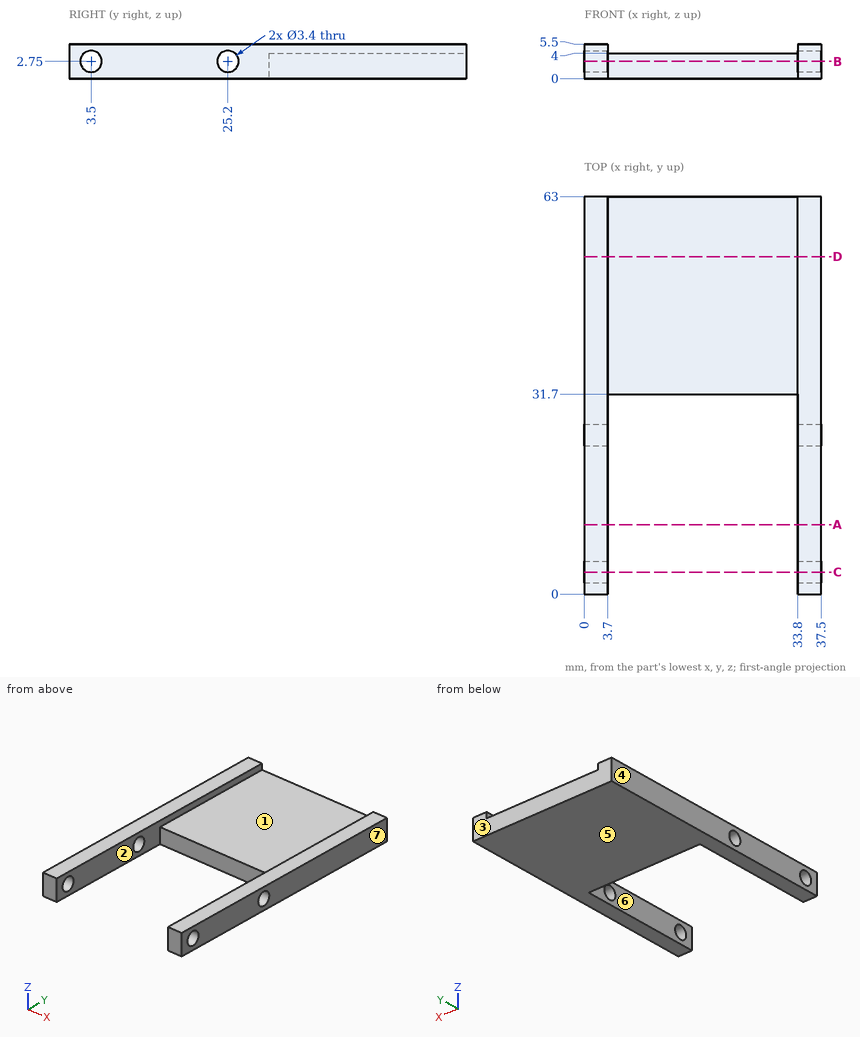
The figure shows three views and two pictorial views of one solid part (mm, origin at its lowest corner). Answer the questions. A direction names the side the tool comes from. Give positions to 0.01 mm unless a question says otherwise; leave off trailing zeros. Write each loop counter-clockwise with the first axis right and the second up, starting at its lowest first coordinate (ties: lowest second). Pieces come first, ordered by that corner, then holes. Notation, with made-up numbers: M 69.25,85 L 78.25,85 A21 ccw 78.25,105 Z; hole C 75.5,-18.5 d8. An arc over 180 degrees is marked long. One line per item, written item: value. Start each with the question number.
(1) Find section D-D (y = 53.5). Determine the outline of the cut face in (x, z).
(2) Determine the mould class of the marked faces 4, 5, 6 and 7 for opening direction X: pulls with the +X half, pulls with the -X half, needs draft (parallel to the pull), parting line crosses it, or undercut.
(3) Flat-ended cylindrical pins translate along their axes: pin 1 Ø15 at (x, y) = (12.5, 43.5) entering from +Z; pin 2 Ø1.2 at (x, z) = (26, 2) entering from -Y. Find the tip coordinate at first contact, or state that the pin passes through.
(4) Find the intervals of material crossed by line 1 (Y direction, x = 2.75, z = 2.75); line 2 (X direction, y = 19.5, z = 4.9); line 3 (Z direction, x = 2, y = 25), in increasing order.
(5) Find section A-A (y = 11). Determine the outline of the cut face in (x, z), plus the area to 3 significant figures.
(6) Find section C-C (y = 3.5). Determine the outline of the cut face in (x, z).
(7) Find section B-B (z = 2.75). Determine the outline of the cut face in (x, y), plus the area to 3 significant figures.
(8) A tool of negligible diameter and unlimited length cuts with its end or side. For the marked faces 1, 2 and 3, from which of +Z, -Z, +X, -X, +Y, -Y can it reach the whole face along a straight path? Write none if from no direction.
Results below:
1. outline: M 0,0 L 37.5,0 L 37.5,5.5 L 33.8,5.5 L 33.8,4 L 3.7,4 L 3.7,5.5 L 0,5.5 Z
2. face 4: pulls with the -X half
2. face 5: needs draft
2. face 6: undercut
2. face 7: pulls with the +X half
3. pin 1: stops at z = 4
3. pin 2: stops at y = 31.7
4. line 1: y = 0 to 1.8, 5.2 to 23.5, 26.9 to 63
4. line 2: x = 0 to 3.7, 33.8 to 37.5
4. line 3: z = 0 to 1.06, 4.44 to 5.5
5. outline: M 0,0 L 3.7,0 L 3.7,5.5 L 0,5.5 Z; M 33.8,0 L 37.5,0 L 37.5,5.5 L 33.8,5.5 Z
5. area: 40.7 mm^2
6. outline: M 0,0 L 3.7,0 L 3.7,1.05 L 0,1.05 Z; M 0,4.45 L 3.7,4.45 L 3.7,5.5 L 0,5.5 Z; M 33.8,0 L 37.5,0 L 37.5,1.05 L 33.8,1.05 Z; M 33.8,4.45 L 37.5,4.45 L 37.5,5.5 L 33.8,5.5 Z
7. outline: M 0,0 L 3.7,0 L 3.7,1.8 L 0,1.8 Z; M 0,5.2 L 3.7,5.2 L 3.7,23.5 L 0,23.5 Z; M 0,26.9 L 3.7,26.9 L 3.7,31.7 L 33.8,31.7 L 33.8,26.9 L 37.5,26.9 L 37.5,63 L 0,63 Z; M 33.8,0 L 37.5,0 L 37.5,1.8 L 33.8,1.8 Z; M 33.8,5.2 L 37.5,5.2 L 37.5,23.5 L 33.8,23.5 Z
7. area: 1,360 mm^2
8. face 1: +Z, +Y, -Y
8. face 2: +Z, -Y
8. face 3: +Z, -Z, +X, -X, +Y
